Verification items for this drawing (mm, ordinates from the low corner). A direction names the side the tool comes from. Round coordinates to 2 decimals unless told otherwise and drop trailing zeros. Order: outer loops, then holes, each group sorted by start corner. A loop starts at its lowest first (then second) coordinate and runs counter-clockwise, first axis right, second up. Notation, with made-up numbers: (82.25, -10.5) -> (87.25, -10.5) arc R14 cw to (87.25, -2.5) -> close; hole circle Ø10 at (73.25, 10). An arc over 180 degrees is marked (long way). Answer in a Markdown table with one row per item. Add a question column.
1. Sectioned sample at D-D, the plane z = 7. Record the boundary of the cut face in (x, y).
2. Depth check by flat-ended pin: P1, Ø2, axis at y = 9.14, z = 6.5, coming from the -X side; P2, Ø0.8, axis at x = 2, y = 5.5, coming from the -Z side; P3, Ø1.6, axis at x = 0.5, y = 9.5, coming from the +Z side; P4, Ø1.5, axis at y = 3.5, z = 5.5, coming from the -X side. Enter the tip coordinate at first touch or a pass-through.
3. Access from +Z, -Z, +X, -X, +Y, -Y to the whole of each face (thin tool, end or side, straight path). Record for the marked faces 5, 6, 7, 8 and 9.
4. Sectioned sample at B-B, the plane x = 1. Record the boundary of the cut face in (y, z), then the cut area to 3 significant figures.
5. Sectioned sample at A-A, the plane x = 2. Record the boundary of the cut face in (y, z).
6. Draft check along Y on the marked faces 1, 2, 3 and 4. Enter one of: +Y half, -Y half, draft (parallel to the pull), parting line (faces both ways), or undercut.
7. Material ranges on L1, parallel to Y at x = 2.5, z = 6.5; L2, parallel to Y at x = 1.75, z = 1.5; L3, parallel to Y at x = 2.15, z = 6, recorded low to high. Write a range as from..to.
8. Sectioned sample at C-C, the plane z = 2. Record the boundary of the cut face in (x, y).
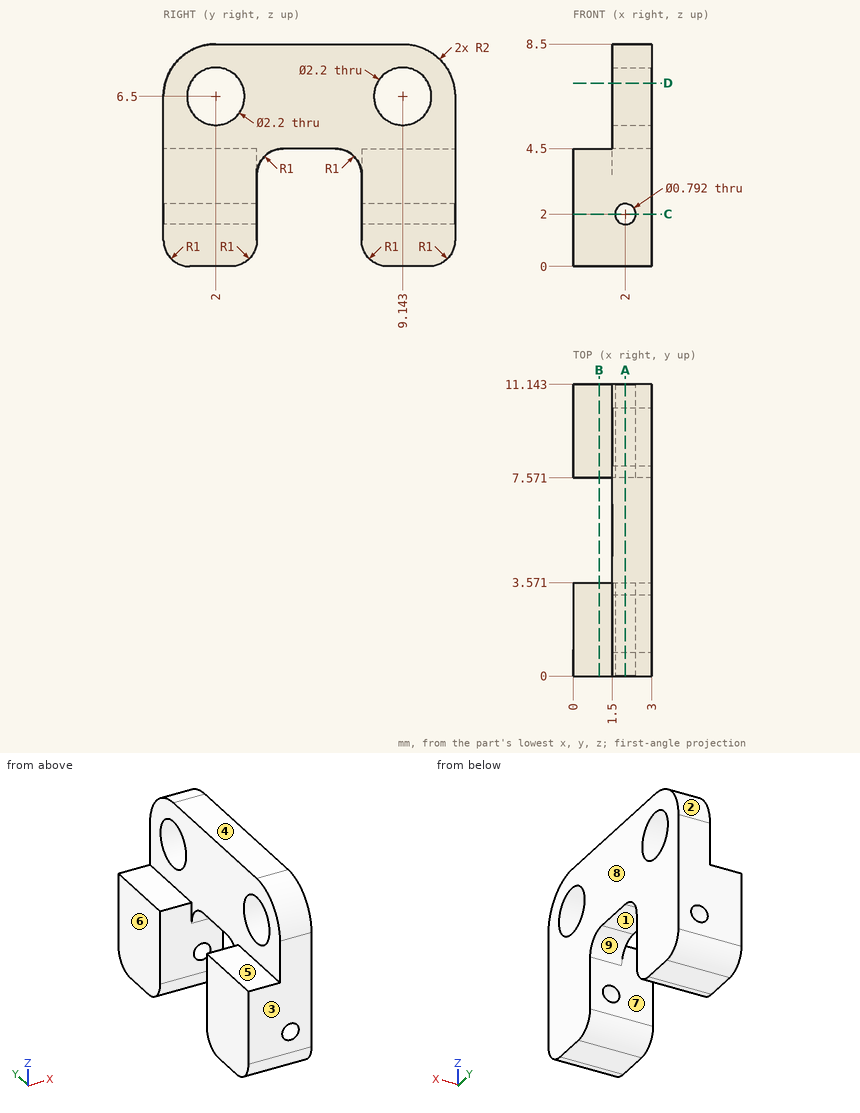
Answer key:
| question | item | result |
|---|---|---|
| 1 | outline | (1.5, 0.06) -> (3, 0.06) -> (3, 1.02) -> (1.5, 1.02) -> close; (1.5, 2.98) -> (3, 2.98) -> (3, 8.16) -> (1.5, 8.16) -> close; (1.5, 10.12) -> (3, 10.12) -> (3, 11.08) -> (1.5, 11.08) -> close |
| 2 | P1 | passes through |
| 2 | P2 | stops at z = 4.5 |
| 2 | P3 | stops at z = 4.5 |
| 2 | P4 | stops at x = 1.5 |
| 3 | face 5 | +Z, -X, +Y, -Y |
| 3 | face 6 | +Z, -Z, -X, +Y, -Y |
| 3 | face 7 | -Z, -X |
| 3 | face 8 | +Z, -Z, +X, +Y, -Y |
| 3 | face 9 | -Z, +X, -X |
| 4 | outline | (0, 1) arc R1 ccw to (1, 0) -> (2.57, 0) arc R1 ccw to (3.57, 1) -> (3.57, 4.5) -> (0, 4.5) -> close; (7.57, 1) arc R1 ccw to (8.57, 0) -> (10.14, 0) arc R1 ccw to (11.14, 1) -> (11.14, 4.5) -> (7.57, 4.5) -> close |
| 4 | area | 31.3 mm² |
| 5 | outline | (0, 1) arc R1 ccw to (1, 0) -> (2.57, 0) arc R1 ccw to (3.57, 1) -> (3.57, 1.6) -> (0, 1.6) -> close; (0, 2.4) -> (3.57, 2.4) -> (3.57, 3.5) arc R1 cw to (4.57, 4.5) -> (6.57, 4.5) arc R1 cw to (7.57, 3.5) -> (7.57, 2.4) -> (11.14, 2.4) -> (11.14, 6.5) arc R2 ccw to (9.14, 8.5) -> (2, 8.5) arc R2 ccw to (0, 6.5) -> close; (7.57, 1) arc R1 ccw to (8.57, 0) -> (10.14, 0) arc R1 ccw to (11.14, 1) -> (11.14, 1.6) -> (7.57, 1.6) -> close; hole circle Ø2.2 at (2, 6.5); hole circle Ø2.2 at (9.14, 6.5) |
| 6 | face 1 | undercut |
| 6 | face 2 | +Y half |
| 6 | face 3 | -Y half |
| 6 | face 4 | draft |
| 7 | L1 | y = 0..0.9, 3.1..8.04, 10.24..11.14 |
| 7 | L2 | y = 0..3.57, 7.57..11.14 |
| 7 | L3 | y = 0..1.02, 2.98..8.16, 10.12..11.14 |
| 8 | outline | (0, 0) -> (1.6, 0) -> (1.6, 3.57) -> (0, 3.57) -> close; (0, 7.57) -> (1.6, 7.57) -> (1.6, 11.14) -> (0, 11.14) -> close; (2.4, 0) -> (3, 0) -> (3, 3.57) -> (2.4, 3.57) -> close; (2.4, 7.57) -> (3, 7.57) -> (3, 11.14) -> (2.4, 11.14) -> close |
